from build123d import *

# Parameters (mm, degrees)
F0_R     = 6.5
F1_DEPTH = 3


with BuildPart() as f1:
    # F0 (on Top) → F1 (new body)
    with BuildSketch(Plane.XY):
        with BuildLine():
            ThreePointArc((45.107527, -93.788211), (88.753802, -55.045718), (104.972745, 1.016069))
            ThreePointArc((104.972745, 1.016069), (-56.089042, 89.797126), (-45.162038, -93.788211))
            Line((-45.162038, -93.788211), (-26.15007, -74.776243))
            Line((-26.15007, -74.776243), (26.095559, -74.776243))
            Line((26.095559, -74.776243), (45.107527, -93.788211))
        make_face()
        with Locations((-91.341169, -22.449345)):
            Circle(F0_R, mode=Mode.SUBTRACT)
        with Locations((91.286659, -22.449345)):
            Circle(F0_R, mode=Mode.SUBTRACT)
        Polygon((-85.022339, -10), (-85.022339, 0), (-85.022339, 10), (-10, 10), (-10, 86.016065), (0, 86.016065), (10, 86.016065), (10, 10), (78.260288, 10), (78.260288, 0), (78.260288, -10), align=None, mode=Mode.SUBTRACT)
        with Locations((-29.749685, 90.793084)):
            Circle(F0_R, mode=Mode.SUBTRACT)
        with Locations((29.269962, 90.793084)):
            Circle(F0_R, mode=Mode.SUBTRACT)
    extrude(amount=F1_DEPTH)


solid = f1.part
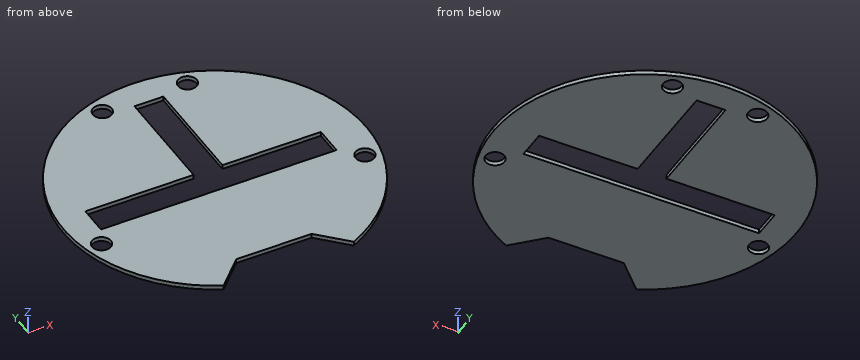
Design review of the part built by this model. Coordinates are the model's own, in mm. Give positions to 0.01 mm unless a question says otherwise; leave off trailing zeros. Order: outer loops, then holes, each group sorted by start corner. A loop starts at its lowest first (then second) coordinate and runs counter-clockwise, first axis right, second up.
1. To check wall thickness, follow L1, parallel to Y at x = -29, z = 2.1; L2, parallel to X at y = 9, z = 1; L3, parallel to X at y = 6.5, z = 2.05. State the ranges of each line that lie inside material, in increasing order.
Solution:
L1: y = -77.63 to -10, 10 to 84.34, 97.25 to 101.94
L2: x = -104.72 to -85.02, 78.26 to 104.67
L3: x = -104.88 to -85.02, 78.26 to 104.83
2. Add section A-A, the plane y = 70.5. State the section outline as (x, z) points.
Solution:
outline: (-78.75, 0) - (-10, 0) - (-10, 3) - (-78.75, 3) - close; (10, 0) - (78.69, 0) - (78.69, 3) - (10, 3) - close
3. For pin 1 Ø11.5 at (x, y) = (-91.34, -22.45) entering from -Z; pin 2 Ø1.5 at (y, z) = (2.5, 1) entering from +X; pin 3 Ø1.5 at (y, z) = (2, 1.5) entering from -X; pin 4 Ø0.9 at (x, z) = (31, 1) entering from +Y, all flat-tipped, find the tip position at first contact; note any pin that passes through.
Solution:
pin 1: passes through
pin 2: stops at x = 104.97
pin 3: stops at x = -105.03
pin 4: stops at y = 101.47
4. Add section B-B, the plane x = -70. State the section outline as (y, z) points, then the cut area to 3 significant figures.
Solution:
outline: (-77.27, 0) - (-10, 0) - (-10, 3) - (-77.27, 3) - close; (10, 0) - (79.3, 0) - (79.3, 3) - (10, 3) - close
area: 410 mm2
5. Add section D-D, the plane y = -60. State the section outline as (x, z) points.
Solution:
outline: (-85.48, 0) - (85.42, 0) - (85.42, 3) - (-85.48, 3) - close
6. Add section C-C, the plane z = 2.45. State the section outline as (x, y) points, then the cut area to 3 significant figures.
Solution:
outline: (-45.16, -93.79) - (-26.15, -74.78) - (26.1, -74.78) - (45.11, -93.79) arc R105 ccw (long way) to start; hole circle Ø13 at (-91.34, -22.45); hole (-85.02, -10) - (78.26, -10) - (78.26, 10) - (10, 10) - (10, 86.02) - (-10, 86.02) - (-10, 10) - (-85.02, 10) - close; hole circle Ø13 at (-29.75, 90.79); hole circle Ø13 at (29.27, 90.79); hole circle Ø13 at (91.29, -22.45)
area: 27,300 mm2
